Work out the finished part from the listing and answer in its coordinate system (mm). A direction names the side the tool comes from. Round coordinates to 2 decimals unless told otherwise and drop trailing zeros. Loops run counter-clockwise (first coordinate to the right, second up) from the corner with the lowest first, then second, coordinate; pieces in that order, holes last. Notation, with made-up numbers: M 46,17.25 L 76,17.25 A26 ccw 76,54.25 Z; hole C 6,17.25 d8. An arc over 180 degrees is marked long. One line per item, written item: value.
```python
from build123d import *

# Parameters (mm, degrees)
BOSS_EXTRUDE1_DEPTH     = 12.7
SKETCH2_R               = 3.2639
CUT_EXTRUDE1_DEPTH      = 4.23
CUT_EXTRUDE1_DEPTH_BACK = 40
SKETCH3_R               = 4
CUT_EXTRUDE2_DEPTH      = 31.75
SKETCH4_W               = 3.1115
SKETCH4_H               = 42.23
BOSS_EXTRUDE2_DEPTH     = 31.75
FILLET4_R               = 1.27


with BuildPart() as part:
    # Sketch1 → Boss-Extrude1 (new body, symmetric)
    with BuildSketch(Plane.XY):
        with BuildLine():
            Line((81.95454797, -39), (81.95454797, -32.65))
            Line((81.95454797, -32.65), (56.55454797, -32.65))
            Line((56.55454797, -32.65), (56.55454797, 3.23))
            Line((56.55454797, 3.23), (24.80454797, 3.23))
            Line((24.80454797, 3.23), (24.80454797, -3.12))
            Line((24.80454797, -3.12), (38.874999678, -3.12))
            ThreePointArc((38.874999678, -3.12), (33.796327751, -19.462996443), (22.209775375, -32.05816398))
            ThreePointArc((22.209775375, -32.05816398), (20.742990597, -36.326618838), (24.379499585, -39))
            Line((24.379499585, -39), (81.95454797, -39))
        make_face()
    extrude(amount=BOSS_EXTRUDE1_DEPTH, both=True)

    # Sketch2 → Cut-Extrude1 (cut, two sides)
    with BuildSketch(Plane(origin=(0, 0, 0), x_dir=(1, 0, 0), z_dir=(0, 1, 0))) as cut_extrude1_sk:
        with Locations((69.25454797, 0)):
            Circle(SKETCH2_R)
    extrude(amount=CUT_EXTRUDE1_DEPTH, mode=Mode.SUBTRACT)
    extrude(cut_extrude1_sk.sketch, amount=-CUT_EXTRUDE1_DEPTH_BACK, mode=Mode.SUBTRACT)

    # Sketch3 → Cut-Extrude2 (cut)
    with BuildSketch(Plane(origin=(0, 3.23, 0), x_dir=(1, 0, 0), z_dir=(0, 1, 0))):
        with Locations((32, 0)):
            Circle(SKETCH3_R)
    extrude(amount=-CUT_EXTRUDE2_DEPTH, mode=Mode.SUBTRACT)

    # Sketch4 → Boss-Extrude2 (add)
    with BuildSketch(Plane.ZY.offset(-24.80454797)):
        with Locations((-11.14425, -17.885)):
            Rectangle(SKETCH4_W, SKETCH4_H)
        with Locations((11.14425, -17.885)):
            Rectangle(SKETCH4_W, SKETCH4_H)
    extrude(amount=-BOSS_EXTRUDE2_DEPTH)

    # Fillet4
    fillet4_edges = [part.edges().sort_by_distance(p)[0] for p in [
        (24.80454797, 3.23, 0),
        (56.55454797, 3.23, 0),
        (56.55454797, -32.65, 0),
        (81.95454797, -32.65, 0),
        (24.80454797, -30.095421579, -11.14425),
        (24.80454797, -30.095421579, 11.14425),
    ]]
    fillet(fillet4_edges, radius=FILLET4_R)


solid = part.part
```
1) Find section B-B (z = 0). Give the number of separate pieces and of enclosed holes in the cut face, then the cut area to 3 significant figures.
Check values:
separate pieces: 3
enclosed holes: 0
area: 1,130 mm2
2) Find section D-D (y = -4.5). Give the vertices of the cut face in (x, z), then the cut area to 3 significant figures.
Check values:
outline: M 24.8,-12.7 L 56.55,-12.7 L 56.55,12.7 L 24.8,12.7 L 24.8,9.59 L 38.74,9.59 L 38.74,-9.59 L 24.8,-9.59 Z
area: 539 mm2
3) Find section A-A (x = 71). Give the vertices of the cut face in (y, z), then the cut area to 3 significant figures.
Check values:
outline: M -39,-12.7 L -32.65,-12.7 L -32.65,-2.76 L -39,-2.76 Z; M -39,2.76 L -32.65,2.76 L -32.65,12.7 L -39,12.7 Z
area: 126 mm2
4) Each of these flat-tipped pins is pushed along its axis until it touches: pin 1 (6.5 mm diameter, centred on x = 32, z = 0, fed in from +Y); pin 2 (10 mm diameter, centred on y = -16.5, z = -5, fed in from -X); pin 3 (7.5 mm diameter, centred on y = -17, z = 0.5, fed in from +X). Where does it stop, or does it pass through?
Check values:
pin 1: y = -28.52
pin 2: x = 24.8
pin 3: x = 56.55
5) Find the intervals of material crossed by probe 1 along X at (y, z) = (-1.25, 0); probe 2 along X at (y, z) = (-12, -11); probe 3 along Y at (x, z) = (30, 5.75), in increasing order. Write a range as from..to.
Check values:
probe 1: 24.8..28, 36..56.55
probe 2: 24.8..56.55
probe 3: -39..-24.92, -3.12..3.23
6) The mould has two halves that part along X. Classify faces 1 (the face through (30, -14, -9.588)), 2 (the face through (81.57, -33.01, 0.18)), 3 (the face through (35.815, -23.168, -1.201)), 4 (the face through (72.368, -35.781, -0.98)): +X half, -X half, draft (parallel to the pull), parting line (faces both ways), or undercut.
Check values:
face 1: draft
face 2: +X half
face 3: undercut
face 4: undercut
7) For faces 5 (the face through (24.805, 0, 0)), 6 (the face through (67, -32.65, 3)), 7 (the face through (35.642, -15.831, 3)), determine the directions among +Z, -Z, +X, -X, +Y, -Y from which every point of the face is accessible in a straight line to the end or side of a thin tool.
Check values:
face 5: +Z, -Z, -X, +Y
face 6: +Z, -Z, +X, +Y
face 7: -X
